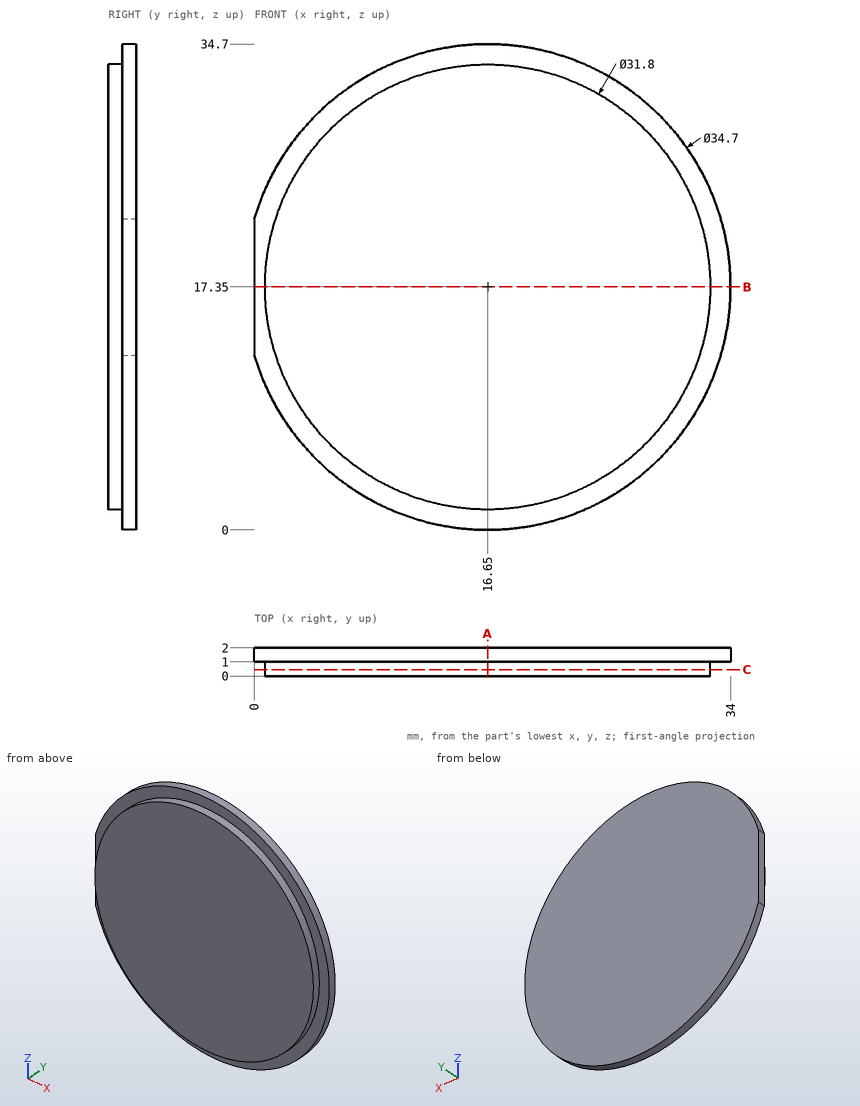
Print and shaded views of the part. All mm, measured from the part's lowest x, y and z. Give positions to 0.01 mm unless a question says otherwise; leave off trailing zeros. Order: outer loops, then holes, each group sorted by start corner. A loop starts at its lowest first (then second) coordinate and runs counter-clockwise, first axis right, second up. Notation, with made-up numbers: M 77,62.5 L 117,62.5 A24 cw 117,88.5 Z; hole C 86,63.25 d2. An arc over 180 degrees is marked long. Use one line per item in the form item = value.
Q1. Slice it at B-B, the plane z = 17.35. Write the cut outline in (x, y).
Conclusion:
outline = M 0,1 L 0.75,1 L 0.75,0 L 32.55,0 L 32.55,1 L 34,1 L 34,2 L 0,2 Z
Q2. Wall check: probe 1 along Y at (x, z) = (17.5, 33.5); probe 2 along X at (y, z) = (1.45, 29.5); probe 3 along X at (y, z) = (0.2, 15). Give the ranges that are in metal, low to high.
Conclusion:
probe_1 = 1 to 2
probe_2 = 4.26 to 29.04
probe_3 = 0.92 to 32.38
Q3. Slice it at A-A, the plane x = 16.65. Write the cut outline in (y, z), and give its area (3 significant figures).
Conclusion:
outline = M 0,1.45 L 1,1.45 L 1,0 L 2,0 L 2,34.7 L 1,34.7 L 1,33.25 L 0,33.25 Z
area = 66.5 mm2
Q4. Slice it at C-C, the plane y = 0.45. Write the cut outline in (x, z), and give its area (3 significant figures).
Conclusion:
outline = C 16.65,17.35 d31.8
area = 794 mm2
Q5. Pin check, flat tips, straight feed: P1, Ø8, axis at x = 14, z = 5, coming from the -Y side; P2, Ø3, axis at x = 30.5, z = 6.5, coming from the -Y side. Stop position of each tip, or through.
Conclusion:
P1 = 0
P2 = 1
